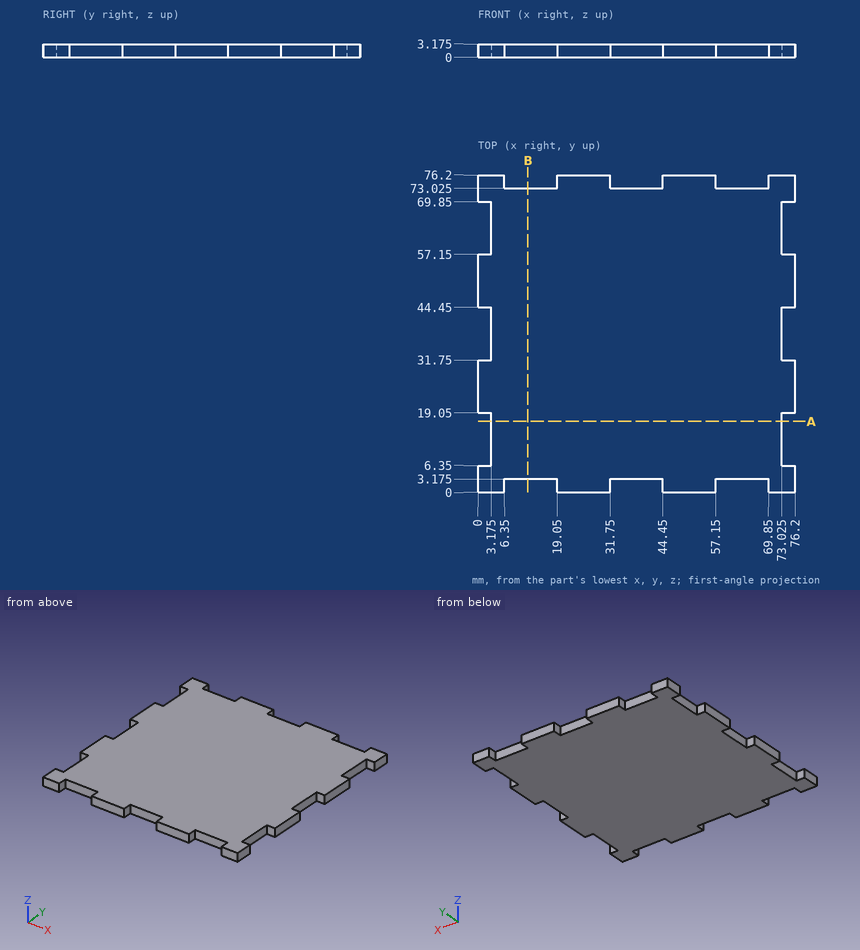
The figure shows three views and two pictorial views of one solid part (mm, origin at its lowest corner). Answer the questions. Round coordinates to 2 decimals unless told otherwise and drop trailing zeros. Order: outer loops, then holes, each group sorted by start corner. A loop starts at its lowest first (then second) coordinate and runs counter-clockwise, first axis right, second up.
Q1. Given pin 1 Ø1 at (x, z) = (62.5, 1) entering from -Y (3 decimals), flat-ended and moving along its own axis, determine where the tip first touches the part or whether it passes through.
Solution:
pin 1: stops at y = 3.175
Q2. Find the intervals of material crossed by line 1 along X through (y, z) = (67, 0.45) (3 decimals), in increasing order.
Solution:
line 1: x = 3.175 to 73.025
Q3. A cutting plane is placed at A-A, the plane y = 17. Determine the outline of the cut face in (x, z) (3 decimals), then the cut area to 3 significant figures.
Solution:
outline: (3.175, 0) - (73.025, 0) - (73.025, 3.175) - (3.175, 3.175) - close
area: 222 mm2
